```python
from build123d import *

# Parameters (mm, degrees)
SKETCH1_R                = 4
BOSS_EXTRUDE1_DEPTH      = 180
M3_CLEARANCE_HOLE1_D     = 3.242
M3_CLEARANCE_HOLE1_DEPTH = 15
M3_CLEARANCE_HOLE1_TIP   = 0.973995063
M3_CLEARANCE_HOLE2_D     = 3.242
M3_CLEARANCE_HOLE2_DEPTH = 15
M3_CLEARANCE_HOLE2_TIP   = 0.973995063
CHAMFER1_SIZE            = 0.5


with BuildPart() as part:
    # Sketch1 → Boss-Extrude1 (new, symmetric)
    with BuildSketch(Plane(origin=(0, 0, 0), x_dir=(0, -1, 0), z_dir=(-1, 0, 0))):
        with Locations(Location((0, 0, 0), (0, 0, 90))):
            Circle(SKETCH1_R)
    extrude(amount=BOSS_EXTRUDE1_DEPTH, both=True)

    # M3 Clearance Hole1
    with Locations(Plane(origin=(180, 0, 0), x_dir=(0, 0, -1), z_dir=(1, 0, 0))):
        with Locations((0, 0)):
            Hole(M3_CLEARANCE_HOLE1_D / 2, depth=M3_CLEARANCE_HOLE1_DEPTH)
            with Locations((0, 0, -(M3_CLEARANCE_HOLE1_DEPTH + M3_CLEARANCE_HOLE1_TIP / 2))):  # 118° drill point
                Cone(0, M3_CLEARANCE_HOLE1_D / 2, M3_CLEARANCE_HOLE1_TIP, mode=Mode.SUBTRACT)

    # M3 Clearance Hole2
    with Locations(Plane.ZY.offset(180)):
        with Locations((0, 0)):
            Hole(M3_CLEARANCE_HOLE2_D / 2, depth=M3_CLEARANCE_HOLE2_DEPTH)
            with Locations((0, 0, -(M3_CLEARANCE_HOLE2_DEPTH + M3_CLEARANCE_HOLE2_TIP / 2))):  # 118° drill point
                Cone(0, M3_CLEARANCE_HOLE2_D / 2, M3_CLEARANCE_HOLE2_TIP, mode=Mode.SUBTRACT)

    # Chamfer1
    chamfer1_edges = [part.edges().sort_by_distance(p)[0] for p in [
        (-180, 0, -4),
        (180, 0, -4),
    ]]
    chamfer(chamfer1_edges, length=CHAMFER1_SIZE)


solid = part.part
```
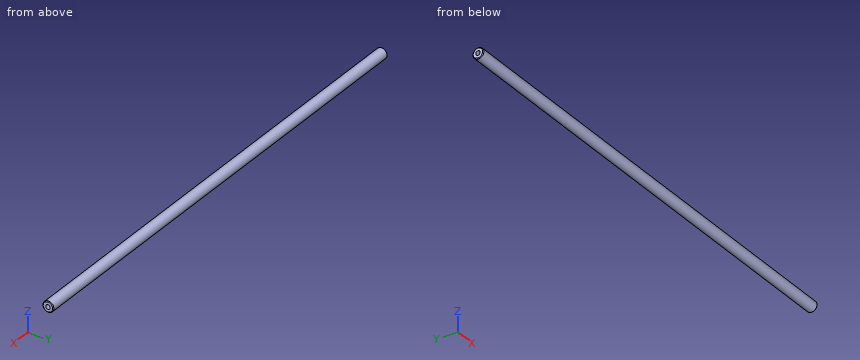
The model under review builds one solid part; all positions refer to its coordinate system, in mm. Coordinates: 2 decimals unless noted, no trailing zeros. Order: outer loops, then holes, each group sorted by start corner. A loop starts at its lowest first (then second) coordinate and runs counter-clockwise, first axis right, second up. Notation, with made-up numbers: (85.5, 12) -> (131.5, 12) arc R28 cw to (131.5, 49) -> close; hole circle Ø3 at (12, -20.75). An arc over 180 degrees is marked (long way). Answer in a Markdown table with one row per item. Add a question column.
Item 1: We need section A-A on x = 140.5. Write out the cut boundary in (y, z), plus the area to 3 significant figures.
Item 2: To check wall thickness, follow probe 1 along Y at (x, z) = (170.5, 0); probe 2 along Y at (x, z) = (24.5, -0.75). State the ranges of each line that lie inside material, in increasing order.
Item 3: Clearance check with a flat-ended pin moving along its axis: pin 1 (4 mm diameter, centred on x = 84.5, z = -2.5, fed in from +Y). State where the tip first meets the part, or that it passes through.
Final values:
| question | item | result |
|---|---|---|
| 1 | outline | circle Ø8 at (0, 0) |
| 1 | area | 50.3 mm2 |
| 2 | probe 1 | y = -4 to -1.62, 1.62 to 4 |
| 2 | probe 2 | y = -3.93 to 3.93 |
| 3 | pin 1 | stops at y = 3.97 |
